from build123d import *

# Parameters (mm, degrees)
SKETCH_1_R               = 120
EXTRUDE_1_DEPTH          = 35
SKETCH_9_R               = 112.5
EXTRUDE_2_DEPTH          = 0.5
SKETCH_6_R               = 112.5
EXTRUDE_3_DEPTH          = 0.5
SKETCH_5_R               = 100
CUT_EXTRUDE_2_DEPTH      = 1.5
CUT_EXTRUDE_2_DEPTH_BACK = 36.5
SKETCH_4_R               = 1.75
CUT_EXTRUDE_3_DEPTH      = 5
SKETCH_2_R               = 1.75
CUT_EXTRUDE_4_DEPTH      = 5
SKETCH_10_R              = 1.6
CUT_EXTRUDE_6_DEPTH      = 6
CUT_EXTRUDE_START        = 36
SKETCH_11_R              = 1.6
CUT_EXTRUDE_7_DEPTH      = 6.5


with BuildPart() as part:
    # Эскиз1 → Бобышка-Вытянуть1 (new body)
    with BuildSketch(Plane.XY):
        Circle(SKETCH_1_R)
    extrude(amount=EXTRUDE_1_DEPTH)

    # Эскиз7 → Вырез-Повернуть2 (revolve, cut)
    with BuildSketch(Plane(origin=(0, 0, 0), x_dir=(1, 0, 0), z_dir=(0, 1, 0))):
        with BuildLine():
            Line((-120, 0), (-120, -4.5))
            Line((-120, -4.5), (-113, -4.5))
            ThreePointArc((-113, -4.5), (-109.464466094, -5.964466094), (-108, -9.5))
            Line((-108, -9.5), (-108, -25.5))
            ThreePointArc((-108, -25.5), (-109.464466094, -29.035533906), (-113, -30.5))
            Line((-113, -30.5), (-120, -30.5))
            Line((-120, -30.5), (-120, -35))
            Line((-120, -35), (-128.220660741, -35))
            Line((-128.220660741, -35), (-128.220660741, 0))
            Line((-128.220660741, 0), (-120, 0))
        make_face()
    revolve(axis=Axis((0, 0, 0), (0, 0, 1)), mode=Mode.SUBTRACT)

    # Эскиз9 → Бобышка-Вытянуть2 (add)
    with BuildSketch(Plane.XY.offset(35)):
        Circle(SKETCH_9_R)
    extrude(amount=EXTRUDE_2_DEPTH)

    # Эскиз6 → Бобышка-Вытянуть3 (add)
    with BuildSketch(Plane(origin=(0, 0, 0), x_dir=(-1, 0, 0), z_dir=(0, 0, -1))):
        Circle(SKETCH_6_R)
    extrude(amount=EXTRUDE_3_DEPTH)

    # Эскиз5 → Вырез-Вытянуть2 (cut, two sides)
    with BuildSketch(Plane.XY.offset(35)) as cut_extrude_2_sk:
        Circle(SKETCH_5_R)
    extrude(amount=CUT_EXTRUDE_2_DEPTH, mode=Mode.SUBTRACT)
    extrude(cut_extrude_2_sk.sketch, amount=-CUT_EXTRUDE_2_DEPTH_BACK, mode=Mode.SUBTRACT)

    # Эскиз4 → Вырез-Вытянуть3 (cut)
    with BuildSketch(Plane.XY.offset(35)):
        with Locations((-115.5, 0)):
            Circle(SKETCH_4_R)
        with Locations((-108.534497701, 39.503326554)):
            Circle(SKETCH_4_R)
        with Locations((-88.47813318, 74.241968919)):
            Circle(SKETCH_4_R)
        with Locations((-57.75, 100.025934137)):
            Circle(SKETCH_4_R)
        with Locations((-20.056364521, 113.745295473)):
            Circle(SKETCH_4_R)
        with Locations((20.056364521, 113.745295473)):
            Circle(SKETCH_4_R)
        with Locations((57.75, 100.025934137)):
            Circle(SKETCH_4_R)
        with Locations((88.47813318, 74.241968919)):
            Circle(SKETCH_4_R)
        with Locations((108.534497701, 39.503326554)):
            Circle(SKETCH_4_R)
        with Locations((115.5, 0)):
            Circle(SKETCH_4_R)
        with Locations((108.534497701, -39.503326554)):
            Circle(SKETCH_4_R)
        with Locations((88.47813318, -74.241968919)):
            Circle(SKETCH_4_R)
        with Locations((57.75, -100.025934137)):
            Circle(SKETCH_4_R)
        with Locations((20.056364521, -113.745295473)):
            Circle(SKETCH_4_R)
        with Locations((-20.056364521, -113.745295473)):
            Circle(SKETCH_4_R)
        with Locations((-57.75, -100.025934137)):
            Circle(SKETCH_4_R)
        with Locations((-88.47813318, -74.241968919)):
            Circle(SKETCH_4_R)
        with Locations((-108.534497701, -39.503326554)):
            Circle(SKETCH_4_R)
    extrude(amount=-CUT_EXTRUDE_3_DEPTH, mode=Mode.SUBTRACT)

    # Эскиз2 → Вырез-Вытянуть4 (cut)
    with BuildSketch(Plane(origin=(0, 0, 0), x_dir=(-1, 0, 0), z_dir=(0, 0, -1))):
        with Locations((0, 115.5)):
            Circle(SKETCH_2_R)
        with Locations((39.503326554, 108.534497701)):
            Circle(SKETCH_2_R)
        with Locations((74.241968919, 88.47813318)):
            Circle(SKETCH_2_R)
        with Locations((100.025934137, 57.75)):
            Circle(SKETCH_2_R)
        with Locations((113.745295473, 20.056364521)):
            Circle(SKETCH_2_R)
        with Locations((113.745295473, -20.056364521)):
            Circle(SKETCH_2_R)
        with Locations((100.025934137, -57.75)):
            Circle(SKETCH_2_R)
        with Locations((74.241968919, -88.47813318)):
            Circle(SKETCH_2_R)
        with Locations((39.503326554, -108.534497701)):
            Circle(SKETCH_2_R)
        with Locations((0, -115.5)):
            Circle(SKETCH_2_R)
        with Locations((-39.503326554, -108.534497701)):
            Circle(SKETCH_2_R)
        with Locations((-74.241968919, -88.47813318)):
            Circle(SKETCH_2_R)
        with Locations((-100.025934137, -57.75)):
            Circle(SKETCH_2_R)
        with Locations((-113.745295473, -20.056364521)):
            Circle(SKETCH_2_R)
        with Locations((-113.745295473, 20.056364521)):
            Circle(SKETCH_2_R)
        with Locations((-100.025934137, 57.75)):
            Circle(SKETCH_2_R)
        with Locations((-74.241968919, 88.47813318)):
            Circle(SKETCH_2_R)
        with Locations((-39.503326554, 108.534497701)):
            Circle(SKETCH_2_R)
    extrude(amount=-CUT_EXTRUDE_4_DEPTH, mode=Mode.SUBTRACT)

    # Эскиз10 → Вырез-Вытянуть6 (cut)
    with BuildSketch(Plane(origin=(0, 0, -0.5), x_dir=(-1, 0, 0), z_dir=(0, 0, -1))):
        with Locations((0, 106)):
            Circle(SKETCH_10_R)
        with Locations((74.953318806, 74.953318806)):
            Circle(SKETCH_10_R)
        with Locations((106, 0)):
            Circle(SKETCH_10_R)
        with Locations((74.953318806, -74.953318806)):
            Circle(SKETCH_10_R)
        with Locations((0, -106)):
            Circle(SKETCH_10_R)
        with Locations((-74.953318806, -74.953318806)):
            Circle(SKETCH_10_R)
        with Locations((-106, 0)):
            Circle(SKETCH_10_R)
        with Locations((-74.953318806, 74.953318806)):
            Circle(SKETCH_10_R)
    extrude(amount=-CUT_EXTRUDE_6_DEPTH, mode=Mode.SUBTRACT)

    # Эскиз11 → Вырез-Вытянуть7 (cut)
    with BuildSketch(Plane.XY.offset(CUT_EXTRUDE_START)):
        with Locations((0, 106)):
            Circle(SKETCH_11_R)
        with Locations((74.953318806, 74.953318806)):
            Circle(SKETCH_11_R)
        with Locations((106, 0)):
            Circle(SKETCH_11_R)
        with Locations((74.953318806, -74.953318806)):
            Circle(SKETCH_11_R)
        with Locations((0, -106)):
            Circle(SKETCH_11_R)
        with Locations((-74.953318806, -74.953318806)):
            Circle(SKETCH_11_R)
        with Locations((-106, 0)):
            Circle(SKETCH_11_R)
        with Locations((-74.953318806, 74.953318806)):
            Circle(SKETCH_11_R)
    extrude(amount=-CUT_EXTRUDE_7_DEPTH, mode=Mode.SUBTRACT)


solid = part.part
Model file for the job. Use its own axes, mm. A direction names the side the tool comes from. Coordinates: 2 decimals unless noted, no trailing zeros. Loops run counter-clockwise (first coordinate to the right, second up) from the corner with the lowest first, then second, coordinate; pieces in that order, holes last. Notation, with made-up numbers: (-22, -15.5) -> (-17, -15.5) arc R9 ccw to (-17, 1.5) -> close; hole circle Ø5 at (41.25, 1.5). An arc over 180 degrees is marked (long way). Use one line per item in the form item = value. Start each with the question number.
(1) Cut at A-A on z = 16.5. Give the cut face in (x, y), and give its area (3 significant figures).
(2) Pull direction Z, two halves, no side cores. Call faces 1 (the flat face through (35, 107.2, 0)), 2 (the flat face through (35, 107.2, 35)), 3 (the cylindrical face through (23.412, 105.432, 17.612)), 4 (the flat face through (-106, 44, 4.5)): pulls with the +Z half, pulls with the -Z half, needs draft (parallel to the pull), parting line crosses it, or undercut.
(3) Tool access for faces 5 (the cylindrical face through (95.38, 30.04, 17.75)), 6 (the cylindrical face through (-112.39, 4.95, 35.25)), 7 (the cylindrical face through (112.39, 4.95, -0.25)), 8 (the flat face through (106, 44, 30.5)): list every direction of +Z, -Z, +X, -X, +Y, -Y with a clear straight run to the whole face (end or side of a thin tool).
(4) Flat gauge pins, fed straight in: pin 1 (4 mm diameter, centred on y = -11, z = 5.5, fed in from -X); pin 2 (8 mm diameter, centred on x = 21.5, z = 22, fed in from -Y); pin 3 (1 mm diameter, centred on x = -0.5, y = -105.5, fed in from +Z). Where does each tip first touch, or does it go through?
(5) Probe probe 1 along Z at (x, y) = (73, -86); probe 2 along X at (y, z) = (-2.5, 32.5); probe 3 along X at (y, z) = (54.5, 11.5). List the from-to ranges inside material, lowest first. Write a range as from..to.
Values:
q1.outline = circle Ø216 at (0, 0); hole circle Ø200 at (0, 0)
q1.area = 5,230 mm2
q2.face_1 = pulls with the -Z half
q2.face_2 = pulls with the +Z half
q2.face_3 = undercut
q2.face_4 = undercut
q3.face_5 = +Z, -Z
q3.face_6 = +Z
q3.face_7 = -Z
q3.face_8 = none
q4.pin_1 = -119.64
q4.pin_2 = -106.57
q4.pin_3 = 29.5
q5.probe_1 = 0..4.5, 30.5..35
q5.probe_2 = -119.97..-99.97, 99.97..119.97
q5.probe_3 = -93.24..-83.84, 83.84..93.24
